```python
from build123d import *

# Parameters (mm, degrees)
SKETCH3_W               = 60
SKETCH3_H               = 15
SKETCH3_R               = 3.5
BOSS_EXTRUDE1_DEPTH     = 4
SKETCH6_W               = 8
SKETCH6_H               = 15
BOSS_EXTRUDE2_DEPTH     = 10
FILLET2_R               = 1.5
CUT_EXTRUDE1_DEPTH      = 46.370695388
CUT_EXTRUDE1_DEPTH_BACK = 46.370695388
SKETCH7_R               = 1.4


with BuildPart() as part:
    # Sketch3 → Boss-Extrude1 (new body)
    with BuildSketch(Plane(origin=(0, 0, 0), x_dir=(1, 0, 0), z_dir=(0, 1, 0))):
        Rectangle(SKETCH3_W, SKETCH3_H)
        with Locations(Location((-24.5, 0, 0), (0, 0, 270))):
            Circle(SKETCH3_R, mode=Mode.SUBTRACT)
        with Locations(Location((24.5, 0, 0), (0, 0, 270))):
            Circle(SKETCH3_R, mode=Mode.SUBTRACT)
    extrude(amount=BOSS_EXTRUDE1_DEPTH)

    # Sketch6 → Boss-Extrude2 (add)
    with BuildSketch(Plane(origin=(0, 4, 0), x_dir=(1, 0, 0), z_dir=(0, 1, 0))):
        with Locations((-8.5, 0)):
            Rectangle(SKETCH6_W, SKETCH6_H)
    boss_extrude2 = extrude(amount=BOSS_EXTRUDE2_DEPTH)

    # Mirror1: Boss-Extrude2 across plane
    add(boss_extrude2.mirror(Plane(origin=(0, 0, 0), x_dir=(0, 0, 1), z_dir=(1, 0, 0))))

    # Fillet2
    fillet2_edges = [part.edges().sort_by_distance(p)[0] for p in [
        (-21.25, 4, 7.5),
        (-21.25, 4, -7.5),
        (0, 4, 7.5),
        (-12.5, 4, 0),
        (-12.5, 9, -7.5),
        (-12.5, 9, 7.5),
        (-4.5, 4, 0),
        (-4.5, 9, 7.5),
        (-4.5, 9, -7.5),
        (-12.5, 14, 0),
        (-8.5, 14, 7.5),
        (-4.5, 14, 0),
        (-8.5, 14, -7.5),
        (21.25, 4, 7.5),
        (0, 4, -7.5),
        (12.5, 14, 0),
        (12.5, 9, 7.5),
        (8.5, 14, -7.5),
        (12.5, 9, -7.5),
        (4.5, 14, 0),
        (4.5, 9, -7.5),
        (8.5, 14, 7.5),
        (4.5, 9, 7.5),
        (12.5, 4, 0),
        (4.5, 4, 0),
        (21.25, 4, -7.5),
    ]]
    fillet(fillet2_edges, radius=FILLET2_R)

    # Sketch7 → Cut-Extrude1 (cut, two sides: drawn at the far end of the back side and taken through both)
    with BuildSketch(Plane.ZY.offset(12.5).offset(-CUT_EXTRUDE1_DEPTH_BACK)):
        with Locations((0, 8.870600297)):
            Circle(SKETCH7_R)
    extrude(amount=CUT_EXTRUDE1_DEPTH + CUT_EXTRUDE1_DEPTH_BACK, mode=Mode.SUBTRACT)


solid = part.part
```
For this review, take the finished solid that the model builds, in its own axes (mm). A direction names the side the tool comes from. Coordinates: 2 decimals unless noted, no trailing zeros. Order: outer loops, then holes, each group sorted by start corner. A loop starts at its lowest first (then second) coordinate and runs counter-clockwise, first axis right, second up. Notation, with made-up numbers: (-38, 79.25) -> (7, 79.25) arc R16 ccw to (7, 103.25) -> close; hole circle Ø8 at (44.25, 5.25). An arc over 180 degrees is marked (long way). Use CSV: the item, a comma, the result in double quotes. Start each with the question number.
Item 1: We need section D-D, the plane z = 4.75. Give the boundary of the cut face in (x, y).
Item 2: For faces 4 (the face through (4.95, 9.05, 7.07)), 5 (the face through (22.11, 3.55, -7.07)), 6 (the face through (-4.07, 4.45, -0.08)), list the 3-axis set-ups (+Z, -Z, +X, -X, +Y, -Y) from which the entire face can be reached by the end or side of a thin tool; tool diameter is ignored.
Item 3: We need section A-A, the plane x = -24.5. Give the boundary of the cut face in (y, z), then the cut area to 3 significant figures.
Item 4: Insertion check: pin 1 (3 mm diameter, centred on x = 14.5, z = -6, fed in from +Y); pin 2 (2.5 mm diameter, centred on y = 8.87, z = 0, fed in from +X); pin 3 (1.5 mm diameter, centred on y = 5.5, z = 5, fed in from +X); pin 4 (7.5 mm diameter, centred on y = 9, z = 0, fed in from +X). Each pin has a flat end and moves straight along its axis. Give the tip position at first contact, or say it passes through.
Item 5: We need section B-B, the plane x = 8. Give the boundary of the cut face in (y, z).
Item 6: Wall thickness on probe 1 along X at (y, z) = (3.25, 0); probe 2 along X at (y, z) = (7.25, -4.5); probe 3 along Y at (x, z) = (-10, 0): over which ranges is each line inside the solid? List them lowest first.
Item 7: We need section C-C, the plane z = -2.5. Give the boundary of the cut face in (x, y).
Item 8: Draft analysis for pull direction Y (two halves, no side actions). For faces 1 (the face through (4.95, 9.05, -7.07)), 2 (the face through (4.05, 4.43, -0.08)), 3 (the face through (-8.444, 7.504, -0.303)), state which applies: pulls with the +Y half, pulls with the -Y half, needs draft (parallel to the pull), parting line crosses it, or undercut.
Derived:
1,outline,"(-30, 0) -> (30, 0) -> (30, 4) -> (14, 4) arc R1.5 cw to (12.5, 5.5) -> (12.5, 12.5) arc R1.5 ccw to (11, 14) -> (6, 14) arc R1.5 ccw to (4.5, 12.5) -> (4.5, 5.5) arc R1.5 cw to (3, 4) -> (-3, 4) arc R1.5 cw to (-4.5, 5.5) -> (-4.5, 12.5) arc R1.5 ccw to (-6, 14) -> (-11, 14) arc R1.5 ccw to (-12.5, 12.5) -> (-12.5, 5.5) arc R1.5 cw to (-14, 4) -> (-30, 4) -> close"
2,face 4,"+Z, +Y"
2,face 5,"-Z, +X, +Y"
2,face 6,"+Z, -Z, +Y"
3,outline,"(0, -7.5) -> (2.5, -7.5) arc R1.5 ccw to (4, -6) -> (4, -3.5) -> (0, -3.5) -> close; (0, 3.5) -> (4, 3.5) -> (4, 6) arc R1.5 ccw to (2.5, 7.5) -> (0, 7.5) -> close"
3,area,"31.0 mm^2"
4,pin 1,"stops at y = 4.38"
4,pin 2,"passes through"
4,pin 3,"stops at x = 12.7"
4,pin 4,"stops at x = 12.52"
5,outline,"(0, -7.5) -> (12.5, -7.5) arc R1.5 ccw to (14, -6) -> (14, 6) arc R1.5 ccw to (12.5, 7.5) -> (0, 7.5) -> close; hole circle Ø2.8 at (8.87, 0)"
6,probe 1,"x = -30 to -28, -21 to 21, 28 to 30"
6,probe 2,"x = -12.5 to -4.5, 4.5 to 12.5"
6,probe 3,"y = 0 to 7.47, 10.27 to 14"
7,outline,"(-30, 0) -> (-26.95, 0) -> (-26.95, 4) -> (-30, 4) -> close; (-22.05, 0) -> (22.05, 0) -> (22.05, 4) -> (14, 4) arc R1.5 cw to (12.5, 5.5) -> (12.5, 12.5) arc R1.5 ccw to (11, 14) -> (6, 14) arc R1.5 ccw to (4.5, 12.5) -> (4.5, 5.5) arc R1.5 cw to (3, 4) -> (-3, 4) arc R1.5 cw to (-4.5, 5.5) -> (-4.5, 12.5) arc R1.5 ccw to (-6, 14) -> (-11, 14) arc R1.5 ccw to (-12.5, 12.5) -> (-12.5, 5.5) arc R1.5 cw to (-14, 4) -> (-22.05, 4) -> close; (26.95, 0) -> (30, 0) -> (30, 4) -> (26.95, 4) -> close"
8,face 1,"needs draft"
8,face 2,"pulls with the +Y half"
8,face 3,"undercut"
